```python
from build123d import *

# Parameters (mm, degrees)
F1_DEPTH = 20
F6_DEPTH = 16.8440384213


# Not quite as in the source:
# - a pattern or mirror of a feature is missing from the dataset's text; its kind, count and spacing are read off the source's solid
# - a feature names something its author has since deleted; it is built from what else it names


with BuildPart() as f1:
    # F0 (on Front) → F1 (new body, symmetric)
    with BuildSketch(Plane.XZ):
        Polygon((0, 30), (0, 0), (50, 0), (50, 20), align=None)
    extrude(amount=F1_DEPTH, both=True)

    # F5 (on 3pt) → F6 (cut, through all)
    with BuildSketch(Plane(origin=(11.3475177305, -14.1843971631, 28.3687943262), x_dir=(0.9415544714, 0.1506487154, -0.3012974309), z_dir=(-0.3368607684, 0.4210759605, -0.8421519211))):
        Polygon((41.0517749549, 13.416407865), (-12.0518972345, 4.472135955), (41.0517749549, -8.94427191), align=None)
    f6 = extrude(amount=-F6_DEPTH, mode=Mode.SUBTRACT)

    # F6_copies: F6 across plane
    add(f6.mirror(Plane.ZX), mode=Mode.SUBTRACT)

    # F8: sweep along a path in F7
    with BuildLine(Plane(origin=(0, 0, 0), x_dir=(0, -1, 0), z_dir=(-1, 0, 0))) as f8_path:
        Line((20, 30), (20, 40))
    # F1_face1 (on face) → F8 (sweep)
    with BuildSketch(Plane(origin=(16.6666666667, 0, 26.6666666667), x_dir=(1, 0, 0), z_dir=(0.1961161351, 0, 0.9805806757))):
        Polygon((-16.996731712, -20), (33.993463424, 0), (-16.996731712, 20), align=None)
    sweep(path=f8_path.line)


solid = f1.part
```
The listing builds one solid part. Answer for the finished solid, in the listing's coordinates (mm). A direction names the side the tool comes from. Coordinates: 2 decimals unless noted, no trailing zeros. Loops run counter-clockwise (first coordinate to the right, second up) from the corner with the lowest first, then second, coordinate; pieces in that order, holes last. Notation, with made-up numbers: (31, 80) -> (83, 80) arc R8 ccw to (83, 89) -> close; hole circle Ø5 at (79, -1). An arc over 180 degrees is marked (long way). Return JSON: item names as keys, results as strings. Group by question number.
(1) Which of the six approach directions +Z, -Z, +X, -X, +Y, -Y give full straight-line access (tool end or side, diameter ignored) to faces 1 (the flat face through (25, 10, 30)), 2 (the flat face through (25, -10, 30)), 3 (the flat face through (19.09, 0.28, 36.18))?
(2) A cutting plane is placed at A-A on x = 36.5. Write down the section's boundary in (y, z), and give its area (3 significant figures).
(3) A cutting plane is placed at B-B on z = 23. Write down the section's boundary in (x, y).
(4) Find the intervals of material crossed by probe 1 along Z at (x, y) = (25.5, -1); probe 2 along Z at (x, y) = (32, 18); probe 3 along Y at (x, z) = (24.5, 25.5), in increasing order. Write a range as from..to.
(5) A cutting plane is placed at D-D on x = 14. Write down the section's boundary in (y, z), and give its area (3 significant figures).
(6) Given pin 1 Ø10 at (y, z) = (-6.5, 17) entering from +X; pin 2 Ø4 at (x, z) = (37, 26.5) entering from -Y; pin 3 Ø2 at (x, z) = (34, 26) entering from -Y, each flat-ended and moving along its own axis, determine where each tip first touches the part or whether it passes through.
(7) A cutting plane is placed at C-C on y = 7.5. Write down the section's boundary in (x, z), and give its area (3 significant figures).
The answers:
{
 "1": {"face 1": "+Z, +X, +Y", "face 2": "+Z, +X, -Y", "face 3": "+Z, +X, +Y, -Y"},
 "2": {"outline": "(-20, 0) -> (20, 0) -> (20, 15.4) -> (5.4, 22.7) -> (5.4, 32.7) -> (-5.4, 32.7) -> (-5.4, 22.7) -> (-20, 15.4) -> close", "area": "909 mm^2"},
 "3": {"outline": "(0, -20) -> (17.5, -20) -> (35, -6) -> (50, 0) -> (35, 6) -> (17.5, 20) -> (0, 20) -> close"},
 "4": {"probe 1": "z = 0..34.9", "probe 2": "z = 0..18.2", "probe 3": "y = -10.2..10.2"},
 "5": {"outline": "(-20, 0) -> (20, 0) -> (20, 24.4) -> (14.4, 27.2) -> (14.4, 37.2) -> (-14.4, 37.2) -> (-14.4, 27.2) -> (-20, 24.4) -> close", "area": "1,360 mm^2"},
 "6": {"pin 1": "stops at x = 50", "pin 2": "stops at y = -6", "pin 3": "stops at y = -6.8"},
 "7": {"outline": "(0, 0) -> (50, 0) -> (50, 16.25) -> (31.25, 23.75) -> (31.25, 33.75) -> (0, 40) -> close", "area": "1,530 mm^2"}
}
